Part print with two shaded views. Sizes in mm from the minimum x, y, z corner. Coordinates: 2 decimals unless noted, no trailing zeros. Loops run counter-clockwise (first coordinate to the right, second up) from the corner with the lowest first, then second, coordinate; pieces in that order, holes last.
(1) Flat gauge pin, fed straight in: P1, Ø4, axis at x = 83.5, z = 9.5, coming from the -Y side. Where does the tip first touch, or does it go through?
(2) Slice it at C-C (x = 68). Give the cut face in (y, z), and give its area (3 significant figures).
(3) Slice it at D-D (z = 9.5). Give the cut face in (x, y).
(4) Wall check: L1, parallel to Z at x = 83.5, y = 1.45; L2, parallel to Z at x = 74.5, y = 1.35; L3, parallel to X at y = 0.35, z = 22. Give the ranges that are in metal, low to high.
(5) Slice it at A-A (z = 18.5). Give the cut face in (x, y), and give its area (3 significant figures).
(6) Slice it at B-B (x = 8.5). Give the cut face in (y, z), and give its area (3 significant figures).
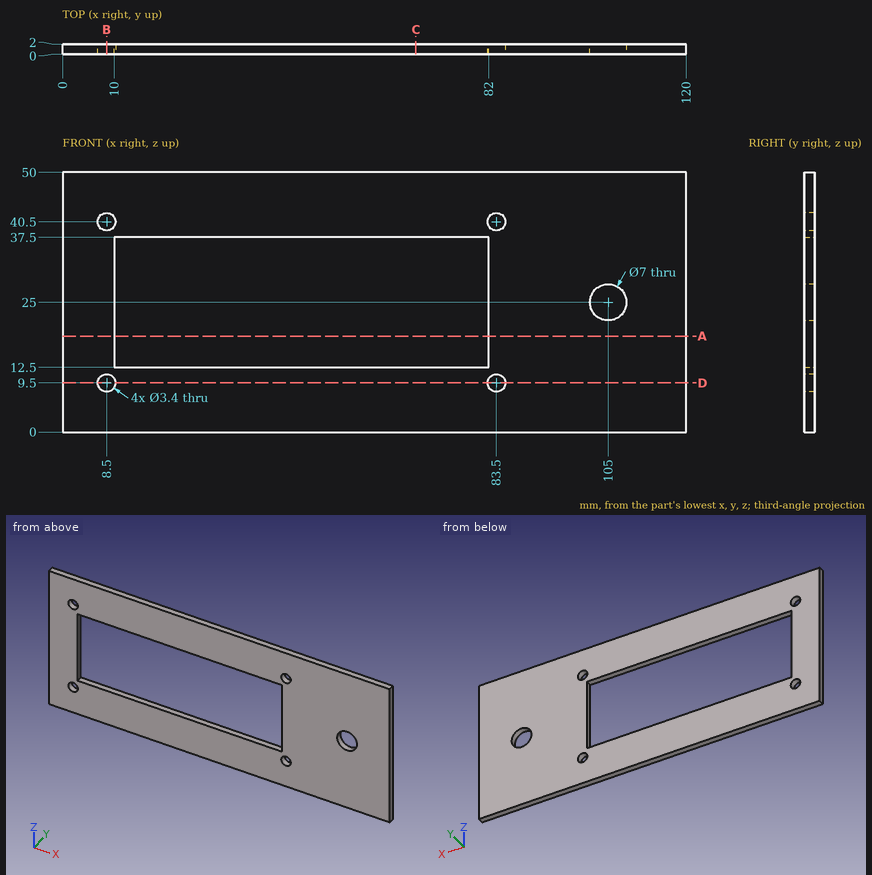
Response values:
1. P1: stops at y = 0
2. outline: (0, 0) - (2, 0) - (2, 12.5) - (0, 12.5) - close; (0, 37.5) - (2, 37.5) - (2, 50) - (0, 50) - close
2. area: 50.0 mm2
3. outline: (0, 0) - (6.8, 0) - (6.8, 2) - (0, 2) - close; (10.2, 0) - (81.8, 0) - (81.8, 2) - (10.2, 2) - close; (85.2, 0) - (120, 0) - (120, 2) - (85.2, 2) - close
4. L1: z = 0 to 7.8, 11.2 to 38.8, 42.2 to 50
4. L2: z = 0 to 12.5, 37.5 to 50
4. L3: x = 0 to 10, 82 to 103.2, 106.8 to 120
5. outline: (0, 0) - (10, 0) - (10, 2) - (0, 2) - close; (82, 0) - (120, 0) - (120, 2) - (82, 2) - close
5. area: 96.0 mm2
6. outline: (0, 0) - (2, 0) - (2, 7.8) - (0, 7.8) - close; (0, 11.2) - (2, 11.2) - (2, 38.8) - (0, 38.8) - close; (0, 42.2) - (2, 42.2) - (2, 50) - (0, 50) - close
6. area: 86.4 mm2
